Source: CAD feature listing. Evaluate the final solid. Frame: model axes, mm. A direction names the side the tool comes from. Give positions to 0.01 mm unless a question says otherwise; leave off trailing zeros. Write each loop counter-clockwise with the first axis right and the second up, starting at its lowest first coordinate (ties: lowest second). Pieces come first, ordered by that corner, then holes. Notation, with made-up numbers: (40.5, 31.5) -> (79.5, 31.5) arc R18 ccw to (79.5, 48.5) -> close; hole circle Ø8 at (-27.5, 38). An arc over 180 degrees is marked (long way). Use a Markdown table: item, result. Add a question column.
```python
from build123d import *

# Parameters (mm, degrees)
F0_W     = 16.5
F0_H     = 36
F1_DEPTH = 4
F2_W     = 10
F2_H     = 30
F3_DEPTH = 30
F4_SIZE  = 9.99999


# Not quite as in the source:
# - a fillet or chamfer is up to 0.001 mm smaller than in the source, because OpenCascade refuses the exact size


with BuildPart() as f1:
    # F0 (on Top) → F1 (new body)
    with BuildSketch(Plane.XY):
        with Locations((8.25, 18)):
            Rectangle(F0_W, F0_H)
    extrude(amount=F1_DEPTH)

    # F2 (on Top) → F3 (join)
    with BuildSketch(Plane.XY):
        with Locations((8.25, 18)):
            Rectangle(F2_W, F2_H)
    extrude(amount=F3_DEPTH)

    # F4 (size 10 in the source; OpenCascade refuses exactly that, so slightly less here)
    f4_edges = [f1.edges().sort_by_distance(p)[0] for p in [
        (3.25, 18, 30),
    ]]
    chamfer(f4_edges, length=F4_SIZE)


solid = f1.part
```
(1) Material intervals for L1, parallel to Z at x = 2, y = 6; L2, parallel to Y at x = 13, z = 22.75; L3, parallel to X at y = 11, z = 7.25, sorted ascending.
(2) Cut plane B-B on x = 12.25. Return the cut outline in (y, z).
(3) Cut plane D-D on x = 6.25. Return the cut outline in (y, z), then the cut area to 3 significant figures.
(4) First-contact query: pin 1 Ø1 at (y, z) = (30, 9) entering from -X; pin 2 Ø1.5 at (x, z) = (12.5, 23) entering from -Y; pin 3 Ø3 at (x, y) = (11.5, 15) entering from +Z; pin 4 Ø8 at (y, z) = (13.5, 6) entering from -X. Flat tips, straight axial feed; report the tip coordinate or a pass-through.
(5) Access query for faces 1 (the flat face through (8, 33, 14)), 2 (the flat face through (13.25, 18, 17)), 3 (the flat face through (8, 3, 14)). Directions: +Z, -Z, +X, -X, +Y, -Y. A direction counts if a zero-diameter tool reaches every point of the face in a straight line with its end or side. Return the directions, or none.
(6) Cut plane C-C on z = 11.25. Return the cut outline in (x, y).
Output:
| question | item | result |
|---|---|---|
| 1 | L1 | 0 to 4 |
| 1 | L2 | 3 to 33 |
| 1 | L3 | 3.25 to 13.25 |
| 2 | outline | (0, 0) -> (36, 0) -> (36, 4) -> (33, 4) -> (33, 29) -> (3, 29) -> (3, 4) -> (0, 4) -> close |
| 3 | outline | (0, 0) -> (36, 0) -> (36, 4) -> (33, 4) -> (33, 23) -> (3, 23) -> (3, 4) -> (0, 4) -> close |
| 3 | area | 714 mm^2 |
| 4 | pin 1 | x = 3.25 |
| 4 | pin 2 | y = 3 |
| 4 | pin 3 | z = 29.75 |
| 4 | pin 4 | x = 0 |
| 5 | face 1 | +Z, +X, -X, +Y |
| 5 | face 2 | +Z, +X, +Y, -Y |
| 5 | face 3 | +Z, +X, -X, -Y |
| 6 | outline | (3.25, 3) -> (13.25, 3) -> (13.25, 33) -> (3.25, 33) -> close |
